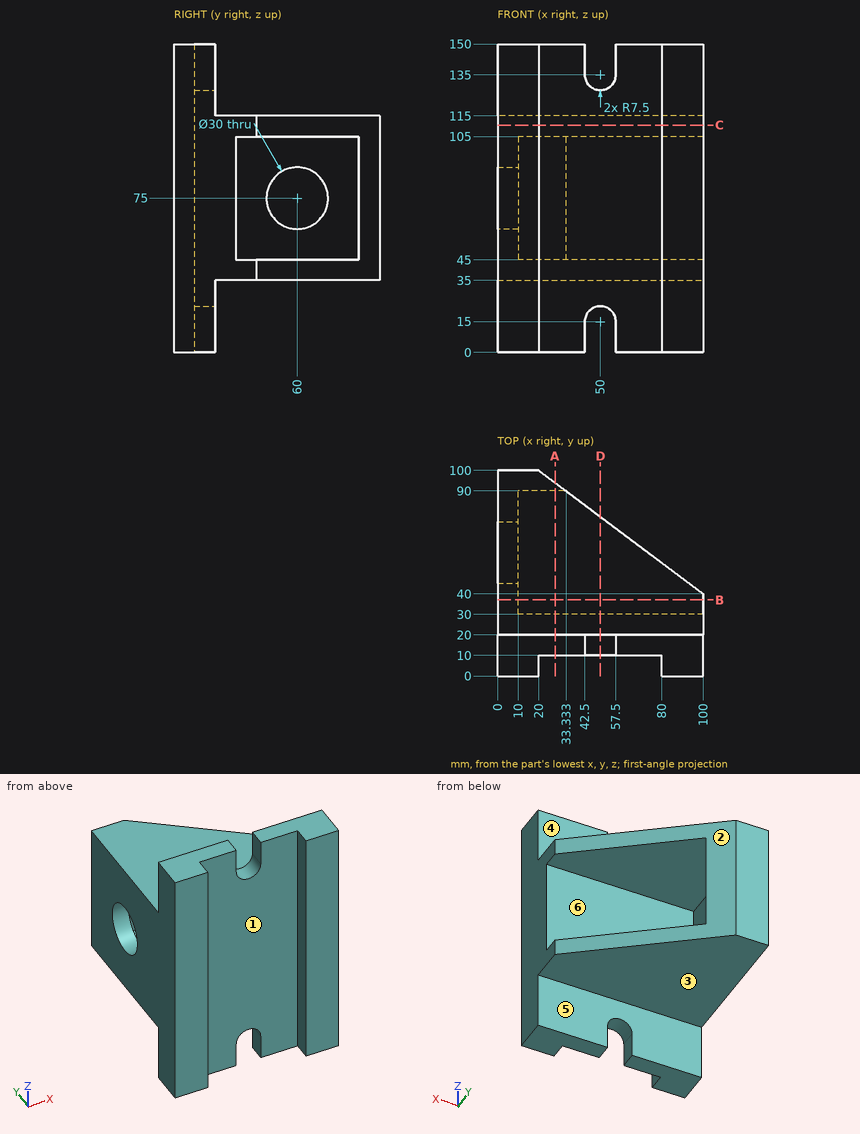
Design review of the part shown in the three views and the two pictorial views. Dimensions are in mm from the part's minimum x, y and z. A direction names the side the tool comes from. Round coordinates to 2 decimals unless told otherwise and drop trailing zeros. Write each loop counter-clockwise with the first axis right and the second up, starting at its lowest first coordinate (ties: lowest second). Pieces come first, ordered by that corner, then holes.
1) Take a section at D-D on x = 50. Give the boundary of the cut face in (y, z).
Answer below:
outline: (10, 22.5) - (20, 22.5) - (20, 35) - (77.5, 35) - (77.5, 45) - (30, 45) - (30, 105) - (77.5, 105) - (77.5, 115) - (20, 115) - (20, 127.5) - (10, 127.5) - close
2) Take a section at C-C on z = 110.5. Give the boundary of the cut face in (x, y).
Answer below:
outline: (0, 0) - (20, 0) - (20, 10) - (80, 10) - (80, 0) - (100, 0) - (100, 40) - (20, 100) - (0, 100) - close
3) For line 1 along Y through (x, z) = (6.75, 75); line 2 along Z through (x, y) = (36.5, 51); line 3 along X through (y, z) = (7, 88.5), list the stretches that pass through material, from the lowest coordinate up.
Answer below:
line 1: y = 0 to 45, 75 to 100
line 2: z = 35 to 45, 105 to 115
line 3: x = 0 to 20, 80 to 100
4) Take a section at B-B on y = 37. Give the boundary of the cut face in (x, z).
Answer below:
outline: (0, 35) - (100, 35) - (100, 45) - (10, 45) - (10, 105) - (100, 105) - (100, 115) - (0, 115) - close
5) Machinability: for the marked faces 4, 5 and 6, which of the approach directions +Z, -Z, +X, -X, +Y, -Y give a long, thin tool a straight path to every point of the face, cutting with its end or side? Answer none if there is none.
Answer below:
face 4: +Z, +X, -X, +Y
face 5: -Z, +X, -X, +Y
face 6: +X
6) Mouldability with a two-part tool opening along X and no side actions: class the marked faces 1, 2 and 3 as +X half, -X half, draft (parallel to the pull), parting line (faces both ways), or undercut.
Answer below:
face 1: undercut
face 2: +X half
face 3: draft
7) Take a section at A-A on x = 28. Give the boundary of the cut face in (y, z).
Answer below:
outline: (10, 0) - (20, 0) - (20, 35) - (94, 35) - (94, 115) - (20, 115) - (20, 150) - (10, 150) - close; hole (30, 45) - (90, 45) - (90, 105) - (30, 105) - close
8) Insertion check: pin 1 Ø24 at (x, y) = (70, 78) entering from +Z; pin 2 Ø6 at (x, z) = (59, 30.5) entering from +Y; pin 3 Ø1.5 at (x, y) = (59.5, 55.5) entering from +Z; pin 4 Ø12 at (x, z) = (50.5, 40.5) entering from +Y (1 decimal). Each pin has a flat end and moves straight along its axis. Give the tip position at first contact, or say it passes through.
Answer below:
pin 1: passes through
pin 2: stops at y = 20
pin 3: stops at z = 115
pin 4: stops at y = 81.6
